Model file for the job. Use its own axes, mm. Round coordinates to 2 decimals unless told otherwise and drop trailing zeros. Loops run counter-clockwise (first coordinate to the right, second up) from the corner with the lowest first, then second, coordinate; pieces in that order, holes last. Notation, with made-up numbers: (73, 76.25) - (128, 76.25) arc R23 ccw to (128, 109.25) - close; hole circle Ø11 at (-30, 54). An arc over 180 degrees is marked (long way). Use one line per item in the form item = value.
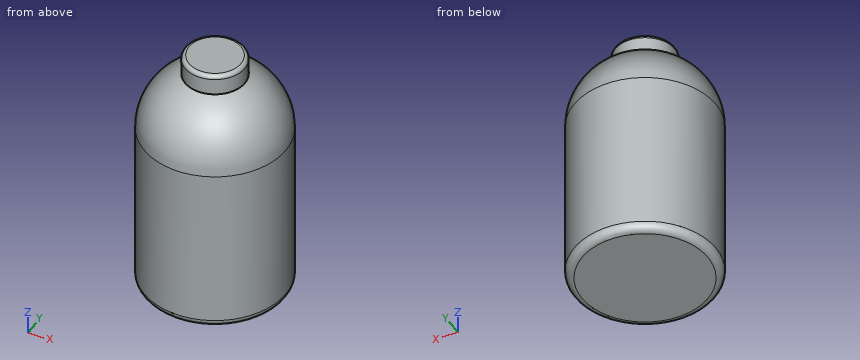
Autodesk Inventor part; units mm, degrees
ref_plane "YZ Plane" through (0, 0, 0) normal (1, 0, 0) x (0, 1, 0)
ref_plane "XZ Plane" through (0, 0, 0) normal (0, 1, 0) x (-1, 0, 0)
ref_plane "XY Plane" through (0, 0, 0) normal (0, 0, 1) x (1, 0, 0)
sketch "Sketch1" plane through (0, 0, 0) normal (0, 0, 1) x (1, 0, 0)
  circle A0 centre (0, 0) radius 9
  dimension "d0" = 18
extrude "Extrusion1" add sketch "Sketch1" along normal blind 30
fillet "Fillet1" radius 8.35 1 edges at (-9, 0, 30)
sketch "Sketch2" plane through (0, 0, 30) normal (0, 0, 1) x (1, 0, 0)
  circle A0 centre (0, 0) radius 3.8
  dimension "d4" = 7.6
extrude "Extrusion2" add sketch "Sketch2" along normal blind 2 and the other way blind 1
fillet "Fillet2" radius 1 1 edges at (-9, 0, 0)
fillet "Fillet3" radius 0.5 1 edges at (-3.8, 0, 32)
properties part number "4g_CO2_Cartridge"
1. Wall check: probe 1 along Y at (x, z) = (-4.75, 26.5); probe 2 along X at (y, z) = (-6.75, 6); probe 3 along Y at (x, z) = (-4, 1). Give the ranges that are in metal, low to high.
Geometry check:
probe_1 = -5.74 to 5.74
probe_2 = -5.95 to 5.95
probe_3 = -8.06 to 8.06
2. Flat gauge pins, fed straight in: pin 1 (1.5 mm diameter, centred on x = -4.5, z = 16.5, fed in from -Y); pin 2 (3 mm diameter, centred on x = -4.5, y = 5, fed in from +Z); pin 3 (5 mm diameter, centred on y = -4, z = 13, fed in from +X). Where does each tip first touch, or does it go through?
Geometry check:
pin_1 = -8.18
pin_2 = 28.63
pin_3 = 8.87
3. Cut at A-A, the plane z = 15. Give the cut face in (x, y).
Geometry check:
outline = circle Ø18 at (0, 0)
